Read the model definition and answer for the solid it produces. Units are mm, in the model's axes. Face numbers are marked on the shaded views. A direction names the side the tool comes from. Round coordinates to 2 decimals unless told otherwise and drop trailing zeros. Answer as CSV lines item,"result".
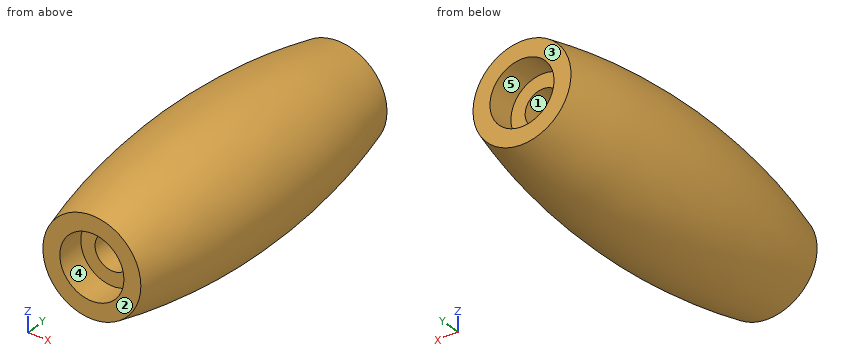
```python
from build123d import *

# Parameters (mm, degrees)
SKETCH_2_R           = 4.5
CUT_EXTRUDE_1_DEPTH  = 49.970922631
EXTRUDE_1_DEPTH      = 19.5
EXTRUDE_1_DEPTH_BACK = 19.5
SKETCH_3_R           = 4.5
SKETCH_3_R_2         = 2.5


with BuildPart() as part:
    # ｽｹｯﾁ1 → 回転1 (revolve)
    with BuildSketch(Plane.XY):
        with BuildLine():
            Line((0, 23.5), (6.882979176, 23.5))
            add(Edge.make_bspline(
                [(6.882979176, -23.5), (12.738297933, 0), (6.882979176, 23.5)],
                knots=[4.373605266, 4.373605266, 4.373605266, 5.051172695, 5.051172695, 5.051172695], degree=2, weights=[1, 0.943159584, 1]))
            Line((6.882979176, -23.5), (0, -23.5))
            Line((0, -23.5), (0, 23.5))
        make_face()
    revolve(axis=Axis((0, 0, 0), (0, 1, 0)))

    # ｽｹｯﾁ2 → ｶｯﾄ - 押し出し1 (cut, through all)
    with BuildSketch(Plane(origin=(0, 23.5, 0), x_dir=(1, 0, 0), z_dir=(0, 1, 0))):
        with Locations(Location((0, 0, 0), (0, 0, 270))):
            Circle(SKETCH_2_R)
    extrude(amount=-CUT_EXTRUDE_1_DEPTH, mode=Mode.SUBTRACT)

    # ｽｹｯﾁ3 → ﾎﾞｽ - 押し出し1 (add, two sides: drawn at the far end of the back side and taken through both)
    with BuildSketch(Plane(origin=(0, 0, 0), x_dir=(1, 0, 0), z_dir=(0, 1, 0)).offset(-EXTRUDE_1_DEPTH_BACK)):
        with Locations(Location((0, 0, 0), (0, 0, 270))):
            Circle(SKETCH_3_R)
        with Locations(Location((0, 0, 0), (0, 0, 270))):
            Circle(SKETCH_3_R_2, mode=Mode.SUBTRACT)
    extrude(amount=EXTRUDE_1_DEPTH + EXTRUDE_1_DEPTH_BACK)


solid = part.part
```
1) Each of these flat-tipped pins is pushed along its axis until it touches: P1, Ø5.5, axis at x = 0, z = 0, coming from the -Y side; P2, Ø6, axis at x = 0, z = 0, coming from the +Y side; P3, Ø4, axis at y = 17.5, z = 2, coming from the -X side; P4, Ø4.5, axis at x = -2, z = 1.5, coming from the -Y side. Where does it stop, or does it pass through?
Evaluation:
P1,"stops at y = -19.5"
P2,"stops at y = 19.5"
P3,"stops at x = -8.41"
P4,"stops at y = -23.5"
2) Straight lines are drawn through the part: line 1 (X direction, y = -22, z = -2.75); line 2 (Z direction, x = -0.75, y = 7); line 3 (X direction, y = -21.95, z = 0). For each, find the intervals that lie inside material, in ascending order.
Evaluation:
line 1,"x = -6.7 to -3.56, 3.56 to 6.7"
line 2,"z = -9.45 to -2.38, 2.38 to 9.45"
line 3,"x = -7.25 to -4.5, 4.5 to 7.25"
3) Determine the mould class of the marked faces 1 and 2 for opening direction Z: released by +Z, released by -Z, zero draft, split by the parting line, or undercut.
Evaluation:
face 1,"undercut"
face 2,"zero draft"
4) A tool of negligible diameter and unlimited length cuts with its end or side. For the marked faces 3, 4 and 5, from which of +Z, -Z, +X, -X, +Y, -Y can it reach the whole face along a straight path? Write none if from no direction.
Evaluation:
face 3,"+Z, -Z, +X, -X, +Y"
face 4,"-Y"
face 5,"+Y"
